Part print with two shaded views. Sizes in mm from the minimum x, y, z corner. A direction names the side the tool comes from. Coordinates: 2 decimals unless noted, no trailing zeros. Order: outer loops, then holes, each group sorted by start corner. A loop starts at its lowest first (then second) coordinate and runs counter-clockwise, first axis right, second up. Notation, with made-up numbers: (6, 76) - (39, 76) arc R21 ccw to (39, 96) - close; hole circle Ø2 at (42.25, 41.25). An arc over 180 degrees is marked (long way). One line per item, written item: value.
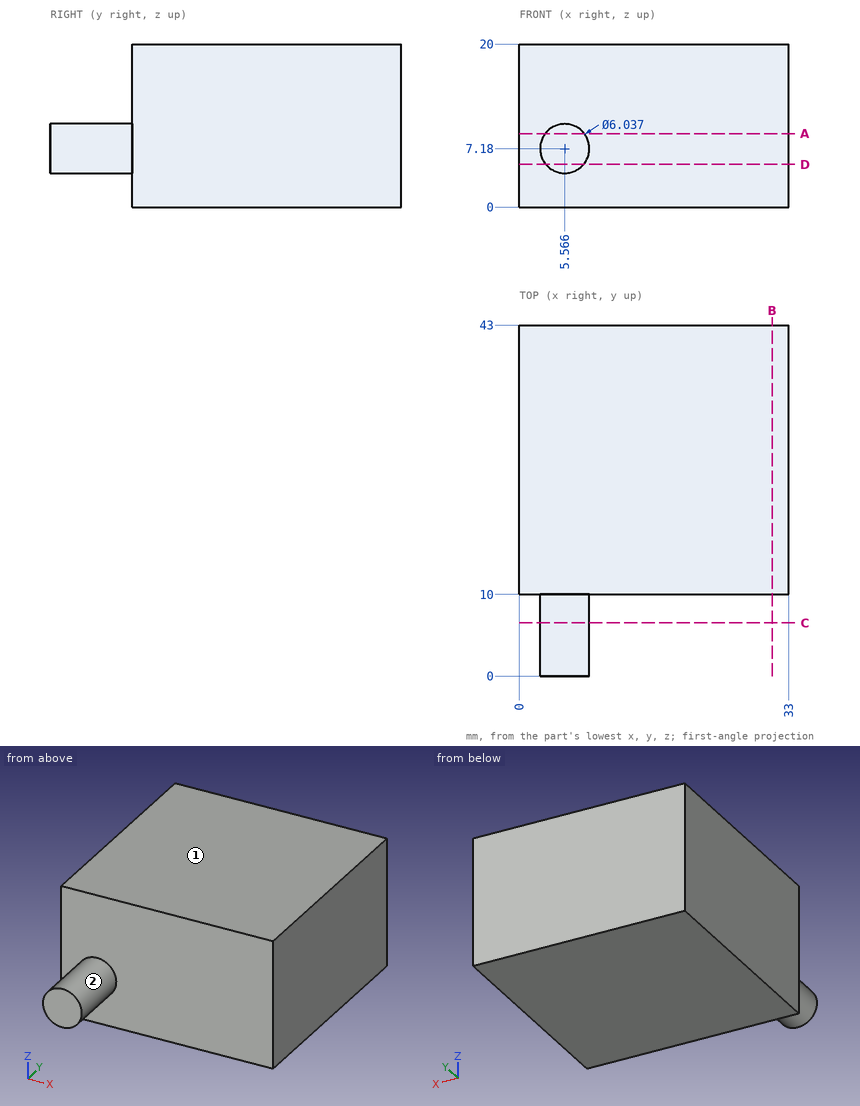
1. Band-saw the part on D-D, the plane z = 5.25. Give the cut face in (x, y) (1 decimal).
Values found:
outline: (0, 10) - (3.2, 10) - (3.2, 0) - (7.9, 0) - (7.9, 10) - (33, 10) - (33, 43) - (0, 43) - close
2. Probe line 1 along Y through (x, z) = (2, 1); line 2 along X through (y, z) = (4.5, 8); line 3 along X through (y, z) = (4, 5.5) (1 decimal). List the from-to ranges inside material, lowest first.
Values found:
line 1: y = 10 to 43
line 2: x = 2.66 to 8.47
line 3: x = 3.1 to 8.1
3. 3-axis set-ups, long thin cutter, end or side, ignore diameter. For the marked faces 1 and 2: which of +Z, -Z, +X, -X, +Y, -Y reach the whole face in a straight line?
Values found:
face 1: +Z, +X, -X, +Y, -Y
face 2: -Y
4. Band-saw the part on C-C, the plane y = 6.5. Give the cut face in (x, z), and give its area (3 significant figures).
Values found:
outline: circle Ø6.04 at (5.57, 7.18)
area: 28.6 mm2
5. Band-saw the part on B-B, the plane x = 31. Give the cut face in (y, z), and give its area (3 significant figures).
Values found:
outline: (10, 0) - (43, 0) - (43, 20) - (10, 20) - close
area: 660 mm2
6. Band-saw the part on A-A, the plane z = 9. Give the cut face in (x, y).
Values found:
outline: (0, 10) - (3.16, 10) - (3.16, 0) - (7.97, 0) - (7.97, 10) - (33, 10) - (33, 43) - (0, 43) - close
7. Flat gauge pin, fed straight in: P1, Ø2, axis at x = 27, z = 9, coming from the -Y side. Where does the tip first touch, or does it go through?
Values found:
P1: stops at y = 10
